Build history of the part. All positions in model axes, mm. A direction names the side the tool comes from. Give positions to 0.01 mm unless a question says otherwise; leave off trailing zeros. Write each loop counter-clockwise with the first axis right and the second up, starting at its lowest first coordinate (ties: lowest second). Pieces come first, ordered by that corner, then holes. Notation, with made-up numbers: (51.5, 48.5) -> (83.5, 48.5) arc R22 ccw to (83.5, 74.5) -> close; hole circle Ø4 at (53.5, 42.25). An arc over 180 degrees is marked (long way). Put each result on its own line as item: value. Start each with the question number.
Item 1: Flat gauge pins, fed straight in: pin 1 Ø8.5 at (x, z) = (12.7, 15.24) entering from +Y; pin 2 Ø1 at (x, y) = (16.5, 12.5) entering from +Z; pin 3 Ø4 at (x, y) = (9, 6) entering from +Z. Where does each tip first touch, or does it go through?
Item 2: Slice it at A-A, the plane x = 12.7. Give the number of separate pieces and of enclosed holes in the cut face, plus the area to 3 significant figures.
Item 3: Drill centre lines: line 1 along X through (y, z) = (2.85, 15.24); line 2 along Z through (x, y) = (18.5, 20.5). Where is each one in solid material? Low to high.
Item 4: Two-plate mould, pull along Y, no slides. Class faces 1 (the cylindrical face through (12.522, 3.388, 24.096)), 2 (the cylindrical face through (9.44, 15.38, 2.41)), 3 (the flat face through (0, 7, 4)): pulls with the +Y half, pulls with the -Y half, needs draft (parallel to the pull), parting line crosses it, or undercut.
Item 5: Slice it at B-B, the plane y = 15.24. List the corners of the cut face in (x, z).
Item 6: Tool access for faces 4 (the flat face through (12.5, 4.762, 11.6)), 5 (the flat face through (25.4, 7, 4)): list every direction of +Z, -Z, +X, -X, +Y, -Y with a clear straight run to the whole face (end or side of a thin tool).
Item 7: Slice it at C-C, the plane z = 17.25. List the corners of the cut face in (x, y), plus the area to 3 significant figures.
```python
from build123d import *

# Parameters (mm, degrees)
BOSS_EXTRUDE1_DEPTH     = 25.4
F_1_4_CLEARANCE_HOLE1_D = 6.5278
F_1_4_CLEARANCE_HOLE2_D = 6.5278


with BuildPart() as part:
    # Sketch1 → Boss-Extrude1 (new body)
    with BuildSketch(Plane(origin=(0, -22.225, 0), x_dir=(0, -1, 0), z_dir=(-1, 0, 0))):
        with BuildLine():
            Line((-22.225, 0), (-22.225, 25.4))
            Line((-22.225, 25.4), (-22.4155, 25.4))
            ThreePointArc((-22.4155, 25.4), (-25.648392204, 24.060892204), (-26.9875, 20.828))
            Line((-26.9875, 20.828), (-26.9875, 7.9375))
            ThreePointArc((-26.9875, 7.9375), (-27.91743597, 5.69243597), (-30.1625, 4.7625))
            Line((-30.1625, 4.7625), (-43.053, 4.7625))
            ThreePointArc((-43.053, 4.7625), (-46.285892204, 3.423392204), (-47.625, 0.1905))
            Line((-47.625, 0.1905), (-47.625, 0))
            Line((-47.625, 0), (-22.225, 0))
        make_face()
    extrude(amount=-BOSS_EXTRUDE1_DEPTH)

    # 1/4 Clearance Hole1 (through all)
    with Locations(Plane(origin=(0, 0, 0), x_dir=(-1, 0, 0), z_dir=(0, 0, -1))):
        with Locations((-12.7, 15.24)):
            Hole(F_1_4_CLEARANCE_HOLE1_D / 2)

    # 1/4 Clearance Hole2 (through all)
    with Locations(Plane(origin=(0, 0, 0), x_dir=(-1, 0, 0), z_dir=(0, -1, 0))):
        with Locations((-12.7, -15.24)):
            Hole(F_1_4_CLEARANCE_HOLE2_D / 2)


solid = part.part
```
Values follow:
1. pin 1: y = 4.76
1. pin 2: z = 4.76
1. pin 3: z = 23.36
2. separate pieces: 3
2. enclosed holes: 0
2. area: 150 mm2
3. line 1: 0 to 9.44, 15.96 to 25.4
3. line 2: 0 to 4.76
4. face 1: pulls with the +Y half
4. face 2: undercut
4. face 3: needs draft
5. outline: (0, 0) -> (9.44, 0) -> (9.44, 4.76) -> (0, 4.76) -> close; (15.96, 0) -> (25.4, 0) -> (25.4, 4.76) -> (15.96, 4.76) -> close
6. face 4: +Z, +X, -X, +Y
6. face 5: +Z, -Z, +X, +Y, -Y
7. outline: (0, 0) -> (10.13, 0) -> (10.13, 4.76) -> (0, 4.76) -> close; (15.27, 0) -> (25.4, 0) -> (25.4, 4.76) -> (15.27, 4.76) -> close
7. area: 96.5 mm2
